Can you work these out from the model? Positions are in its coordinate system, mm. A direction names the side the tool comes from. Coordinates: 2 decimals unless noted, no trailing zeros. Return JSON: item names as keys, results as strings. Group by question number.
```python
from build123d import *

# Parameters (mm, degrees)
SKETCH1_R           = 1.5
BOSS_EXTRUDE1_DEPTH = 2
CHAMFER1_SIZE       = 1
BOSS_EXTRUDE2_DEPTH = 5
SKETCH3_R           = 1.5
SKETCH3_R_2         = 1.654032004
CUT_EXTRUDE1_DEPTH  = 19.458358008


with BuildPart() as part:
    # Sketch1 → Boss-Extrude1 (new body)
    with BuildSketch(Plane.XY):
        with BuildLine():
            Line((8.566894072, -11), (-8.566894072, -11))
            add(Edge.make_bspline(
                [(0, 3.774563681), (-1.6213965, 3.815439451), (-6.14281173, -0.719191195), (-7.529582221, -6.667664167), (-8.566894072, -11)],
                knots=[0, 0, 0, 0, 0.251062994, 1, 1, 1, 1], degree=3))
            add(Edge.make_bspline(
                [(0, 3.774563681), (1.6213965, 3.815439451), (6.14281173, -0.719191195), (7.529582221, -6.667664167), (8.566894072, -11)],
                knots=[0, 0, 0, 0, 0.251062994, 1, 1, 1, 1], degree=3))
        make_face()
        Circle(SKETCH1_R, mode=Mode.SUBTRACT)
    extrude(amount=BOSS_EXTRUDE1_DEPTH)

    # Chamfer1
    chamfer1_edges = [part.edges().sort_by_distance(p)[0] for p in [
        (-1.5, 0, 2),
    ]]
    chamfer(chamfer1_edges, length=CHAMFER1_SIZE)

    # Sketch2 → Boss-Extrude2 (add)
    with BuildSketch(Plane.XY.offset(2)):
        with BuildLine():
            Line((-8.082865754, -9), (8.082865754, -9))
            add(Edge.make_bspline(
                [(8.566894072, -11), (8.407698636, -10.33511982), (8.248472773, -9.667349813), (8.082865754, -9)],
                knots=[0, 0, 0, 0, 0.114938775, 0.114938775, 0.114938775, 0.114938775], degree=3))
            Line((8.566894072, -11), (-8.566894072, -11))
            add(Edge.make_bspline(
                [(-8.082865754, -9), (-8.248472773, -9.667349813), (-8.407698636, -10.33511982), (-8.566894072, -11)],
                knots=[0.885061225, 0.885061225, 0.885061225, 0.885061225, 1, 1, 1, 1], degree=3))
        make_face()
    extrude(amount=BOSS_EXTRUDE2_DEPTH)

    # Sketch3 → Cut-Extrude1 (cut, through all)
    with BuildSketch(Plane.XZ.offset(11)):
        with Locations((-3.566894072, 4.5)):
            Circle(SKETCH3_R)
        with Locations((3.566894072, 4.5)):
            Circle(SKETCH3_R_2)
    extrude(amount=-CUT_EXTRUDE1_DEPTH, mode=Mode.SUBTRACT)


solid = part.part
```
1) If we mould it in two halves opening along Y, with no side actions, what happens to faces 3 (the face through (-1.5, 0.07, 0.49)), 4 (the face through (0, -5, 0)), 5 (the face through (0, -11, 3))? For each: +Y half, -Y half, draft (parallel to the pull), parting line (faces both ways), or undercut.
2) If I drill on line 1 (Z direction, x = -3.5, y = -10); line 2 (X direction, y = -9.5, z = 3.5); line 3 (X direction, y = -9.5, z = 3.75), over which ranges is the centre line in solid material (lowest first)? Write a range as from..to.
3) Suppose I cut it at A-A, the plane z = 4.5. Give the number of separate pieces and of enclosed holes in the cut face, then the cut area to 3 significant figures.
4) For faces 1 (the face through (0, -4, 2)), 2 (the face through (4.33, -10.014, 3.033)), which set-ups out of +Z, -Z, +X, -X, +Y, -Y let a thin tool reach every point of the face, with its end or its side?
5) For pin 1 (4 mm diameter, centred on x = 0.5, z = 4.5, fed in from +Y); pin 2 (4 mm diameter, centred on y = -1, z = 4.5, fed in from +X); pin 3 (3 mm diameter, centred on y = -7, z = 2, fed in from +X); pin 4 (3 mm diameter, centred on y = -4, z = 1, fed in from +X), each with a flat end and sliding along its axis, tell me the tip position at first contact or that it passes through.
Returned:
{
 "1": {"face 3": "undercut", "face 4": "draft", "face 5": "-Y half"},
 "2": {"line 1": "z = 0..3, 6..7", "line 2": "x = -8.21..-4.68, -2.45..2.25, 4.88..8.21", "line 3": "x = -8.21..-4.87, -2.27..2.09, 5.04..8.21"},
 "3": {"separate pieces": "3", "enclosed holes": "0", "area": "20.7 mm²"},
 "4": {"face 1": "+Z, +X, -X, +Y", "face 2": "+Y, -Y"},
 "5": {"pin 1": "stops at y = -9", "pin 2": "passes through", "pin 3": "stops at x = 7.96", "pin 4": "stops at x = 7.12"}
}
